Could you check a few things on this model? Use its own coordinates, in mm. Face numbers are marked on the shaded views. A direction names the side the tool comes from. Give positions to 0.01 mm unless a question says otherwise; leave off trailing zeros. Use one line per item in the form item = value.
from build123d import *

# Parameters (mm, degrees)
F2_W     = 126.1226348579
F2_H     = 41.0738363862
F2_W_2   = 95.882229507
F2_H_2   = 28.761270456
F3_DEPTH = 25.4
F4_R     = 1.5
F5_DEPTH = 2.54


with BuildPart() as f1:
    # F0 (on Top) → F1 (revolve)
    with BuildSketch(Plane.XY):
        with BuildLine():
            Line((0, -17.7920795977), (0, 15.1420421898))
            add(Edge.make_bspline(
                [(0, 15.1420421898), (-3.3266345491, 15.1660395685), (-10.3432012836, 15.2166550499), (-16.9798857885, 3.2507688533), (-17.4681972374, 0.1800565782), (-14.1186973605, -10.5597484182), (-7.7260639278, -14.8351312564), (-2.5986913336, -16.7974986441), (0, -17.7920795977)],
                knots=[0, 0, 0, 0, 0.1810593521, 0.3818919716, 0.4880171584, 0.6735828531, 0.8345629472, 1, 1, 1, 1], degree=3))
        make_face()
    revolve(axis=Axis((0, -1.3250187039, 0), (0, -1, 0)))

    # F2 (on Front) → F3 (cut, symmetric)
    with BuildSketch(Plane.XZ):
        with Locations((5.4968688637, -20.5369181931)):
            Rectangle(F2_W, F2_H)
        with Locations((1.9811727107, 28.830869589)):
            Rectangle(F2_W_2, F2_H_2)
    extrude(amount=F3_DEPTH, both=True, mode=Mode.SUBTRACT)

    # F4 (on face) → F5 (join)
    with BuildSketch(Plane.XY.offset(14.450234361)):
        Circle(F4_R)
    extrude(amount=F5_DEPTH)


solid = f1.part
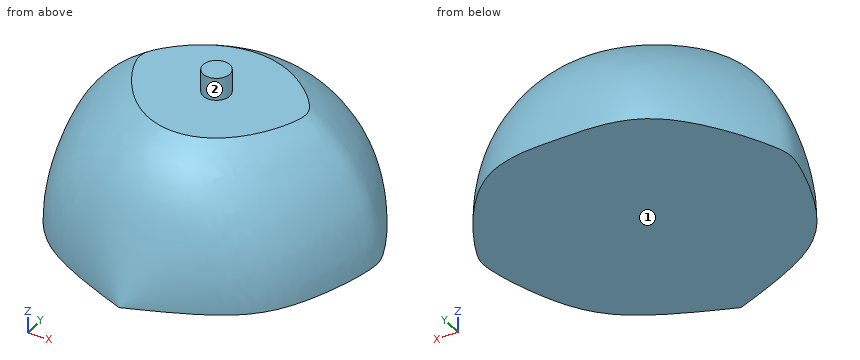
1) For pin 1 Ø8 at (x, y) = (-9, 9) entering from +Z; pin 2 Ø3 at (x, z) = (0, 12) entering from -Y; pin 3 Ø10 at (x, y) = (-11, -8) entering from +Z, each with a flat end and sliding along its axis, tell me the tip position at first contact or that it passes through.
Checked values:
pin_1 = 13.92
pin_2 = -12.78
pin_3 = 14.02
2) If I drill on L1, parallel to Z at x = 2.5, y = -3; L2, parallel to X at y = -8, z = 9.25 (3 decimals); L3, parallel to Y at x = 9.5, z = 12.25, over which ranges is the centre line in solid material (lowest first)?
Checked values:
L1 = 0 to 14.45
L2 = -10.985 to 10.985
L3 = -5.43 to 5.61
3) For the marked faces 1 and 2, which set-ups out of +Z, -Z, +X, -X, +Y, -Y let a thin tool reach every point of the face, with its end or its side?
Checked values:
face_1 = -Z, +X, -X, +Y, -Y
face_2 = +Z
